The model under review builds one solid part; all positions refer to its coordinate system, in mm. Face numbers are marked on the shaded views. A direction names the side the tool comes from. Round coordinates to 2 decimals unless told otherwise and drop trailing zeros. Write each loop counter-clockwise with the first axis right and the second up, starting at its lowest first coordinate (ties: lowest second). Pieces come first, ordered by that corner, then holes. Notation, with made-up numbers: M 49.5,45.25 L 85.5,45.25 A17 ccw 85.5,49.25 Z; hole C -19,75 d2. An arc over 180 degrees is marked long. One line per item, written item: value. Start each with the question number.
1) Wall thickness on probe 1 along Z at (x, y) = (113.5, -129.5); probe 2 along Y at (x, z) = (93.25, -34.5); probe 3 along X at (y, z) = (-31, -27) (3 decimals): over which ranges is each line inside the solid? List them lowest first.
2) Tool access review of the marked faces 1 and 2: name each direction out of +Z, -Z, +X, -X, +Y, -Y from which nothing blocks a thin tool from reaching the whole face with its end or side.
3) Take a section at A-A, the plane y = -162. Write out the cut boundary in (x, z) (3 decimals).
4) For P1, Ø7.5, axis at y = -45, z = -30.5, coming from the -X side (3 decimals); P2, Ø6.5, axis at x = 99, z = -9, coming from the -Y side; P3, Ø6, axis at x = 107.5, y = -73, coming from the +Z side; P4, Ø4.5, axis at x = 100.965, z = -9.525, coming from the -Y side, all flat-tipped, find the tip position at first contact; note any pin that passes through.
from build123d import *

# Parameters (mm, degrees)
EXTRU_MINCE1_DEPTH      = 38.1
ESQUISSE2_R             = 1.89865
ENL_V_MAT_EXTRU_1_DEPTH = 228.663979486
ENL_V_MAT_EXTRU_2_DEPTH = 3.048
D_GAGEMENT_61_D         = 3.7973
ESQUISSE6_W             = 7.62
ESQUISSE6_H             = 267.100210441
ENL_V_MAT_EXTRU_3_DEPTH = 22.86


with BuildPart() as part:
    # Esquisse1 → Extru.-Mince1 (new body)
    with BuildSketch(Plane.XY):
        Polygon((90.805, 44.088736397), (116.205, 44.088736397), (116.205, -223.011474044), (111.125, -223.011474044), (111.125, 39.008736397), (90.805, 39.008736397), align=None)
    extrude(amount=-EXTRU_MINCE1_DEPTH)

    # Esquisse2 → Enlèv. mat.-Extru.1 (cut, through all)
    with BuildSketch(Plane(origin=(116.205, 0, 0), x_dir=(0, 0, -1), z_dir=(1, 0, 0))):
        with Locations(Location((19.05, -202.469224044, 0), (0, 0, 90))):
            Circle(ESQUISSE2_R)
    extrude(amount=-ENL_V_MAT_EXTRU_1_DEPTH, mode=Mode.SUBTRACT)

    # Esquisse3 → Enlèv. mat.-Extru.2 (cut)
    with BuildSketch(Plane.XZ.offset(-39.008736397)):
        Polygon((100.965, -23.735650044), (96.774, -26.155325022), (96.774, -30.994674978), (100.965, -33.414349956), (105.156, -30.994674978), (105.156, -26.155325022), align=None)
        Polygon((100.965, -4.685650044), (96.774, -7.105325022), (96.774, -11.944674978), (100.965, -14.364349956), (105.156, -11.944674978), (105.156, -7.105325022), align=None)
    extrude(amount=-ENL_V_MAT_EXTRU_2_DEPTH, mode=Mode.SUBTRACT)

    # Dégagement #61 (through all)
    with Locations(Plane(origin=(0, 42.056736397, 0), x_dir=(-1, 0, 0), z_dir=(0, -1, 0))):
        with Locations((-100.965, 28.575), (-100.965, 9.525)):
            Hole(D_GAGEMENT_61_D / 2)

    # Esquisse6 → Enlèv. mat.-Extru.3 (cut)
    with BuildSketch(Plane.ZY.offset(-90.805)):
        with Locations((-19.05, -89.461368824)):
            Rectangle(ESQUISSE6_W, ESQUISSE6_H)
    extrude(amount=-ENL_V_MAT_EXTRU_3_DEPTH, mode=Mode.SUBTRACT)


solid = part.part
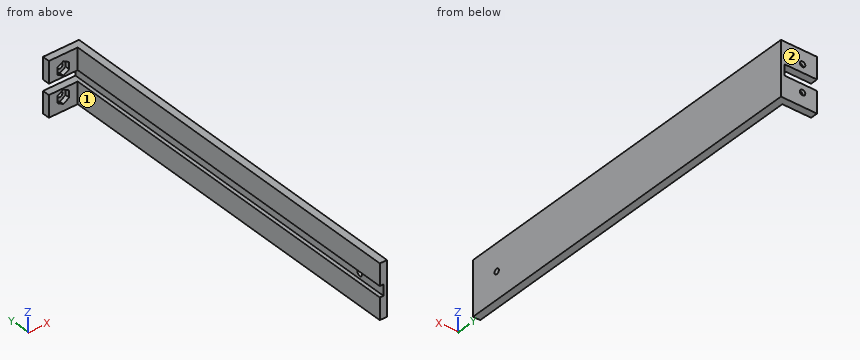
Checked values:
1. probe 1: z = -38.1 to -22.86, -15.24 to 0
1. probe 2: y = 39.01 to 44.09
1. probe 3: x = 111.125 to 116.205
2. face 1: +Z, -Z, -X, -Y
2. face 2: +Z, -Z, +X, -X, +Y
3. outline: M 111.125,-38.1 L 116.205,-38.1 L 116.205,0 L 111.125,0 L 111.125,-15.24 L 113.665,-15.24 L 113.665,-22.86 L 111.125,-22.86 Z
4. P1: stops at x = 111.125
4. P2: stops at y = 39.01
4. P3: passes through
4. P4: stops at y = 42.06
